```python
from build123d import *

# Parameters (mm, degrees)
BOSS_EXTRUDE1_DEPTH      = 11
SHELL1_T                 = -3
SHELL1_THICKNESS_2_DEPTH = 1.5
SKETCH2_R                = 1.3
CUT_EXTRUDE1_DEPTH       = 152
SKETCH3_R                = 1.3
CUT_EXTRUDE2_DEPTH       = 152
CUT_EXTRUDE3_DEPTH       = 152
SKETCH5_W                = 13
SKETCH5_H                = 8
CUT_EXTRUDE4_DEPTH       = 45
FILLET1_R                = 2
CUT_EXTRUDE6_DEPTH       = 92
SKETCH6_R                = 1
CUT_EXTRUDE7_DEPTH       = 5
SKETCH12_R               = 1
CUT_EXTRUDE8_DEPTH       = 5
FILLET2_R                = 1
BOSS_EXTRUDE2_DEPTH      = 11
SKETCH14_R               = 3.1
CUT_EXTRUDE9_DEPTH       = 3.1
CUT_EXTRUDE10_DEPTH      = 9.1
FILLET3_R                = 1
SKETCH19_R               = 1.6
CUT_EXTRUDE12_DEPTH      = 10
FILLET4_R                = 3


with BuildPart() as part:
    # Sketch1 → Boss-Extrude1 (new body)
    with BuildSketch(Plane(origin=(0, 0, 0), x_dir=(1, 0, 0), z_dir=(0, 1, 0))):
        Polygon((38.627416998, 16), (16, 38.627416998), (-16, 38.627416998), (-38.627416998, 16), (-38.627416998, -16), (-16, -38.627416998), (16, -38.627416998), (38.627416998, -16), align=None)
    extrude(amount=BOSS_EXTRUDE1_DEPTH)

    # Shell1
    shell1_openings = [part.faces().sort_by_distance(p)[0] for p in [
        (0, 11, 0),
    ]]
    offset(amount=SHELL1_T, openings=shell1_openings, kind=Kind.INTERSECTION)

    # Shell1 thickness 2 face (on inner face of the shell) → Shell1 thickness 2 (cut)
    with BuildSketch(Plane(origin=(0, 3, 0), x_dir=(0, 0, -1), z_dir=(0, -1, 0))):
        Polygon((-14.757359313, 35.627416998), (14.757359313, 35.627416998), (35.627416998, 14.757359313), (35.627416998, -14.757359313), (14.757359313, -35.627416998), (-14.757359313, -35.627416998), (-35.627416998, -14.757359313), (-35.627416998, 14.757359313), align=None)
    extrude(amount=SHELL1_THICKNESS_2_DEPTH, mode=Mode.SUBTRACT)

    # Sketch2 → Cut-Extrude1 (cut)
    with BuildSketch(Plane(origin=(27.313708499, 0, 27.313708499), x_dir=(0.7071067811865475, 0, -0.7071067811865477), z_dir=(0.7071067811865477, 0, 0.7071067811865475))):
        with Locations((9, 6.75)):
            Circle(SKETCH2_R)
        with Locations((-9, 6.75)):
            Circle(SKETCH2_R)
    extrude(amount=-CUT_EXTRUDE1_DEPTH, mode=Mode.SUBTRACT)

    # Sketch3 → Cut-Extrude2 (cut)
    with BuildSketch(Plane(origin=(-27.313708499, 0, 27.313708499), x_dir=(0.7071067811865476, 0, 0.7071067811865476), z_dir=(-0.7071067811865476, 0, 0.7071067811865476))):
        with Locations((9, 6.75)):
            Circle(SKETCH3_R)
        with Locations((-9, 6.75)):
            Circle(SKETCH3_R)
    extrude(amount=-CUT_EXTRUDE2_DEPTH, mode=Mode.SUBTRACT)

    # Sketch4 → Cut-Extrude3 (cut)
    with BuildSketch(Plane(origin=(38.627416998, 0, 0), x_dir=(0, 0, -1), z_dir=(1, 0, 0))):
        Polygon((0, 1.5), (10, 1.5), (10, 11), (0, 11), (-10, 11), (-10, 1.5), align=None)
    extrude(amount=-CUT_EXTRUDE3_DEPTH, mode=Mode.SUBTRACT)

    # Sketch5 → Cut-Extrude4 (cut)
    with BuildSketch(Plane(origin=(0, 0, -38.627416998), x_dir=(-1, 0, 0), z_dir=(0, 0, -1))):
        with Locations((-6.5, 7)):
            Rectangle(SKETCH5_W, SKETCH5_H)
        with Locations((6.5, 7)):
            Rectangle(SKETCH5_W, SKETCH5_H)
    extrude(amount=-CUT_EXTRUDE4_DEPTH, mode=Mode.SUBTRACT)

    # Fillet1
    fillet1_edges = [part.edges().sort_by_distance(p)[0] for p in [
        (-13, 11, -37.127416998),
        (-13, 3, -37.127416998),
        (13, 11, -37.127416998),
        (13, 3, -37.127416998),
        (37.127416998, 11, 10),
        (37.127416998, 1.5, 10),
        (37.127416998, 11, -10),
        (37.127416998, 1.5, -10),
        (-37.127416998, 11, -10),
        (-37.127416998, 1.5, -10),
        (-37.127416998, 11, 10),
        (-37.127416998, 1.5, 10),
    ]]
    fillet(fillet1_edges, radius=FILLET1_R)

    # Sketch7 → Cut-Extrude6 (cut)
    with BuildSketch(Plane(origin=(0, 1.5, 0), x_dir=(1, 0, 0), z_dir=(0, 1, 0))):
        Polygon((35.627416998, -10.000000003), (31.627416998, -10.000000003), (31.627416998, -18.757359313), (35.627416998, -14.757359313), align=None)
        Polygon((35.627416998, 14.757359313), (35.627416998, 10.000000003), (31.627416998, 10.000000003), (31.627416998, 18.757359313), align=None)
        Polygon((-35.627416998, 10.000000003), (-31.627416998, 10.000000003), (-31.627416998, 18.757359313), (-35.627416998, 14.757359313), align=None)
        Polygon((-35.627416998, -14.757359313), (-35.627416998, -10.000000003), (-31.627416998, -10.000000003), (-31.627416998, -18.757359313), align=None)
    extrude(amount=-CUT_EXTRUDE6_DEPTH, mode=Mode.SUBTRACT)

    # Sketch6 → Cut-Extrude7 (cut)
    with BuildSketch(Plane(origin=(38.627416998, 0, 0), x_dir=(0, 0, -1), z_dir=(1, 0, 0))):
        with Locations((-13, 9.5)):
            Circle(SKETCH6_R)
        with Locations((-13, 2.5)):
            Circle(SKETCH6_R)
        with Locations((13, 2.5)):
            Circle(SKETCH6_R)
        with Locations((13, 9.5)):
            Circle(SKETCH6_R)
    extrude(amount=-CUT_EXTRUDE7_DEPTH, mode=Mode.SUBTRACT)

    # Sketch12 → Cut-Extrude8 (cut)
    with BuildSketch(Plane(origin=(-35.627416998, 0, 0), x_dir=(0, 0, -1), z_dir=(1, 0, 0))):
        with Locations((-13, 9.5)):
            Circle(SKETCH12_R)
        with Locations((-13, 2.5)):
            Circle(SKETCH12_R)
        with Locations((13, 2.5)):
            Circle(SKETCH12_R)
        with Locations((13, 9.5)):
            Circle(SKETCH12_R)
    extrude(amount=-CUT_EXTRUDE8_DEPTH, mode=Mode.SUBTRACT)

    # Fillet2
    fillet2_edges = [part.edges().sort_by_distance(p)[0] for p in [
        (-31.627416998, 0.75, 10.000000003),
        (-31.627416998, 0.75, 18.757359313),
        (-35.627416998, 0.75, 10.000000003),
        (35.627416998, 0.75, -10.000000003),
        (31.627416998, 0.75, -10.000000003),
        (31.627416998, 0.75, -18.757359313),
        (31.627416998, 0.75, 10.000000003),
        (35.627416998, 0.75, 10.000000003),
        (31.627416998, 0.75, 18.757359313),
        (-31.627416998, 0.75, -10.000000003),
        (-35.627416998, 0.75, -10.000000003),
        (-31.627416998, 0.75, -18.757359313),
    ]]
    fillet(fillet2_edges, radius=FILLET2_R)

    # Sketch13 → Boss-Extrude2 (add)
    with BuildSketch(Plane(origin=(0, 11, 0), x_dir=(1, 0, 0), z_dir=(0, 1, 0))):
        Polygon((0, -38.627416998), (-16, -38.627416998), (-14.5, -40.127416998), (0, -40.127416998), align=None)
        Polygon((16, -38.627416998), (0, -38.627416998), (0, -40.127416998), (14.5, -40.127416998), align=None)
    extrude(amount=-BOSS_EXTRUDE2_DEPTH)

    # Sketch14 → Cut-Extrude9 (cut)
    with BuildSketch(Plane.XY.offset(40.127416998)):
        with Locations((8, 3.5)):
            Circle(SKETCH14_R)
        with Locations((-8, 3.5)):
            Circle(SKETCH14_R)
    extrude(amount=-CUT_EXTRUDE9_DEPTH, mode=Mode.SUBTRACT)

    # Sketch18 → Cut-Extrude10 (cut)
    with BuildSketch(Plane.XY.offset(40.127416998)):
        Polygon((-10, 7), (0, 7), (10, 7), (10, 11), (-10, 11), align=None)
    extrude(amount=-CUT_EXTRUDE10_DEPTH, mode=Mode.SUBTRACT)

    # Fillet3
    fillet3_edges = [part.edges().sort_by_distance(p)[0] for p in [
        (-10, 7, 37.877416998),
        (-10, 11, 37.877416998),
        (10, 11, 37.877416998),
        (10, 7, 37.877416998),
    ]]
    fillet(fillet3_edges, radius=FILLET3_R)

    # Sketch19 → Cut-Extrude12 (cut)
    with BuildSketch(Plane(origin=(0, 0, 0), x_dir=(-1, 0, 0), z_dir=(0, -1, 0))):
        Polygon((9, -32.556349186), (9, 32.556349186), (-9, 32.556349186), (-9, -14), (-9, -32.556349186), align=None)
        with Locations(Location((-14, -14, 0), (0, 0, 90))):
            Circle(SKETCH19_R)
        with BuildLine():
            Line((-35.627416998, -11), (-23.627416998, -11))
            ThreePointArc((-23.627416998, -11), (-21.506096654, -10.121320344), (-20.627416998, -8))
            Line((-20.627416998, -8), (-20.627416998, 7.999999998))
            ThreePointArc((-20.627416998, 7.999999998), (-21.506096654, 10.121320342), (-23.627416998, 10.999999998))
            Line((-23.627416998, 10.999999998), (-35.627416998, 10.999999998))
            Line((-35.627416998, 10.999999998), (-35.627416998, -11))
        make_face()
        with BuildLine():
            Line((35.627416998, 11.000000003), (23.627416998, 11.000000003))
            ThreePointArc((23.627416998, 11.000000003), (21.506096652, 10.121320344), (20.627416998, 7.999999997))
            Line((20.627416998, 7.999999997), (20.627416998, -8.000000003))
            ThreePointArc((20.627416998, -8.000000003), (21.506096654, -10.121320346), (23.627416998, -11.000000003))
            Line((23.627416998, -11.000000003), (35.627416998, -11.000000003))
            Line((35.627416998, -11.000000003), (35.627416998, 11.000000003))
        make_face()
        with Locations(Location((14, -14, 0), (0, 0, 90))):
            Circle(SKETCH19_R)
        with Locations(Location((-14, 14, 0), (0, 0, 90))):
            Circle(SKETCH19_R)
        with Locations(Location((14, 14, 0), (0, 0, 90))):
            Circle(SKETCH19_R)
    extrude(amount=-CUT_EXTRUDE12_DEPTH, mode=Mode.SUBTRACT)

    # Fillet4
    fillet4_edges = [part.edges().sort_by_distance(p)[0] for p in [
        (31.627416998, 0.75, -11.000000003),
        (31.627416998, 0.75, 11.000000003),
        (-31.627416998, 0.75, 11.000000003),
        (-31.627416998, 0.75, -11.000000003),
        (-9, 0.75, 32.556349186),
        (9, 0.75, 32.556349186),
        (9, 0.75, -32.556349186),
        (-9, 0.75, -32.556349186),
    ]]
    fillet(fillet4_edges, radius=FILLET4_R)


solid = part.part
```
Input: part model. Units: mm. Frame: model coordinates. A direction names the side the tool comes from. Give positions to 0.01 mm unless a question says otherwise; leave off trailing zeros. Write each loop counter-clockwise with the first axis right and the second up, starting at its lowest first coordinate (ties: lowest second). Pieces come first, ordered by that corner, then holes. Notation, with made-up numbers: (5.5, 63.5) - (60.5, 63.5) arc R19 cw to (60.5, 88.5) - close; hole circle Ø10 at (76, -24.5). An arc over 180 degrees is marked (long way). Write item = value, one per line. Start each with the question number.
1) Pin query (flat end, axial travel): pin 1 (3.5 mm diameter, centred on y = 6, z = -37, fed in from +X); pin 2 (1.5 mm diameter, centred on x = -37.5, z = 0.5, fed in from +Y); pin 3 (1 mm diameter, centred on x = -30.5, y = 7, fed in from -Z). Return the tip coordinate at first contact, or that it passes through.
2) Material intervals for L1, parallel to Y at x = 37, z = -13; L2, parallel to X at y = 1, z = -2.5; L3, parallel to Y at x = -8, z = 37.9, sorted ascending. Write a range as [from, to].
3) Draft query along Z for faces 1 (the face through (0, 7, 38)), 2 (the face through (0, 2, -38.627)), 3 (the face through (-13.93, 0.74, -12.4)). Return one class per face: pulls with the +Z half, pulls with the -Z half, needs draft (parallel to the pull), parting line crosses it, or undercut.
4) Cut plane A-A (z = -7). Return loops of the section in (x, y).
5) Cut plane B-B (x = -1.5). Return loops of the section in (y, z).
6) Reachability of faces 4 (the face through (0, 3, -37)), 5 (the face through (15, 1.5, 0)), 6 (the face through (8.1, 0.8, -31.7)) from +Z, -Z, +X, -X, +Y, -Y: full face, straight path, thin tool, end or side. Return the list, or none.
7) Cut plane C-C (x = 8). Return loops of the section in (y, z), and give its area (3 significant figures).
Answers follow:
q1.pin_1 = 19.38
q1.pin_2 = 1.5
q1.pin_3 = -24.63
q2.L1 = [0, 1.5], [3.5, 8.5], [10.5, 11]
q2.L2 = [-38.63, -35.63], [-20.63, -9], [9, 20.63], [35.63, 38.63]
q2.L3 = [0, 0.4], [6.6, 7]
q3.face_1 = needs draft
q3.face_2 = pulls with the -Z half
q3.face_3 = undercut
q4.outline = (-38.63, 0) - (-35.63, 0) - (-35.63, 1.5) - (-38.63, 1.5) - close; (-20.63, 0) - (-9, 0) - (-9, 1.5) - (-20.63, 1.5) - close; (9, 0) - (20.63, 0) - (20.63, 1.5) - (9, 1.5) - close; (35.63, 0) - (38.63, 0) - (38.63, 1.5) - (35.63, 1.5) - close
q5.outline = (0, -38.63) - (3, -38.63) - (3, -35.63) - (1.5, -35.63) - (1.5, -32.56) - (0, -32.56) - close; (0, 32.56) - (1.5, 32.56) - (1.5, 35.63) - (7, 35.63) - (7, 40.13) - (0, 40.13) - close
q6.face_4 = -Z, +Y
q6.face_5 = +Y
q6.face_6 = +Y, -Y
q7.outline = (0, -38.63) - (3, -38.63) - (3, -35.63) - (1.5, -35.63) - (1.5, -31.79) - (0, -31.79) - close; (0, 31.79) - (1.5, 31.79) - (1.5, 35.63) - (7, 35.63) - (7, 40.13) - (6.6, 40.13) - (6.6, 37.03) - (0.4, 37.03) - (0.4, 40.13) - (0, 40.13) - close
q7.area = 32.8 mm^2
